from build123d import *

# Parameters (mm, degrees)
BOSS_EXTRUDE1_DEPTH = 3.175
SKETCH3_R           = 2.1
CUT_EXTRUDE1_DEPTH  = 4.175


with BuildPart() as part:
    # Sketch1 → Boss-Extrude1 (new body)
    with BuildSketch(Plane(origin=(0, 0, 0), x_dir=(0, 0, -1), z_dir=(1, 0, 0))):
        with BuildLine():
            Line((-62.23, -8.4201), (62.23, -8.4201))
            Line((62.23, -8.4201), (62.23, 8.4201))
            Line((62.23, 8.4201), (-48.006, 8.4201))
            ThreePointArc((-48.006, 8.4201), (-52.493538794, -1.144281181), (-62.23, -5.2451))
            Line((-62.23, -5.2451), (-62.23, -8.4201))
        make_face()
    extrude(amount=BOSS_EXTRUDE1_DEPTH)

    # Sketch3 → Cut-Extrude1 (cut, through all)
    with BuildSketch(Plane.ZY):
        with Locations((-43.18, 2.0701)):
            Circle(SKETCH3_R)
        with Locations((-19.05, 2.0701)):
            Circle(SKETCH3_R)
        with Locations((5.08, 2.0701)):
            Circle(SKETCH3_R)
        with Locations((29.21, 2.0701)):
            Circle(SKETCH3_R)
    extrude(amount=-CUT_EXTRUDE1_DEPTH, mode=Mode.SUBTRACT)


solid = part.part
Geometry check sheet. Reference: the model listing, model coordinates, mm. Give positions to 0.01 mm unless a question says otherwise; leave off trailing zeros. Loops run counter-clockwise (first coordinate to the right, second up) from the corner with the lowest first, then second, coordinate; pieces in that order, holes last. Notation, with made-up numbers: M 13,88 L 46,88 A23 ccw 46,96 Z; hole C -35.5,85.25 d3. An arc over 180 degrees is marked long. Answer as a JSON object with one key per item and string values. Group by question number.
Item 1: Sectioned sample at A-A on z = -19.05. Record the boundary of the cut face in (x, y) (3 decimals), plus the area to 3 significant figures.
Item 2: Sectioned sample at C-C on y = 7.25. Record the boundary of the cut face in (x, z) (3 decimals), plus the area to 3 significant figures.
Item 3: Sectioned sample at B-B on x = 1.15. Record the boundary of the cut face in (y, z), plus the area to 3 significant figures.
Item 4: Sectioned sample at D-D on y = -2.25. Record the boundary of the cut face in (x, z) (3 decimals), plus the area to 3 significant figures.
Item 5: Mould release check, pull along Y, two halves, no side actions. Record for faces 1 (the flat face through (2, -8.42, 1)), 2 (the flat face through (3.175, 0, 1)), 3 (the cylindrical face through (1.57, 0.02, 4.62)): pulls with the +Y half, pulls with the -Y half, needs draft (parallel to the pull), parting line crosses it, or undercut.
Item 6: Material ranges on L1, parallel to Y at x = 2, z = -43.18; L2, parallel to Z at x = 1.15, y = 3.5; L3, parallel to Z at x = 0.2, y = 3.75, recorded low to high.
Findings below:
{
 "1": {"outline": "M 0,-8.42 L 3.175,-8.42 L 3.175,-0.03 L 0,-0.03 Z; M 0,4.17 L 3.175,4.17 L 3.175,8.42 L 0,8.42 Z", "area": "40.1 mm2"},
 "2": {"outline": "M 0,-62.23 L 3.175,-62.23 L 3.175,48.138 L 0,48.138 Z", "area": "350 mm2"},
 "3": {"outline": "M -8.42,-62.23 L 8.42,-62.23 L 8.42,48.01 A14.73 cw -5.25,62.23 L -8.42,62.23 Z; hole C 2.07,-43.18 d4.2; hole C 2.07,-19.05 d4.2; hole C 2.07,5.08 d4.2; hole C 2.07,29.21 d4.2", "area": "1,890 mm2"},
 "4": {"outline": "M 0,-62.23 L 3.175,-62.23 L 3.175,53.786 L 0,53.786 Z", "area": "368 mm2"},
 "5": {"face 1": "pulls with the -Y half", "face 2": "needs draft", "face 3": "undercut"},
 "6": {"L1": "-8.42 to -0.03, 4.17 to 8.42", "L2": "-62.23 to -44.72, -41.64 to -20.59, -17.51 to 3.54, 6.62 to 27.67, 30.75 to 49.24", "L3": "-62.23 to -44.44, -41.92 to -20.31, -17.79 to 3.82, 6.34 to 27.95, 30.47 to 49.13"}
}
